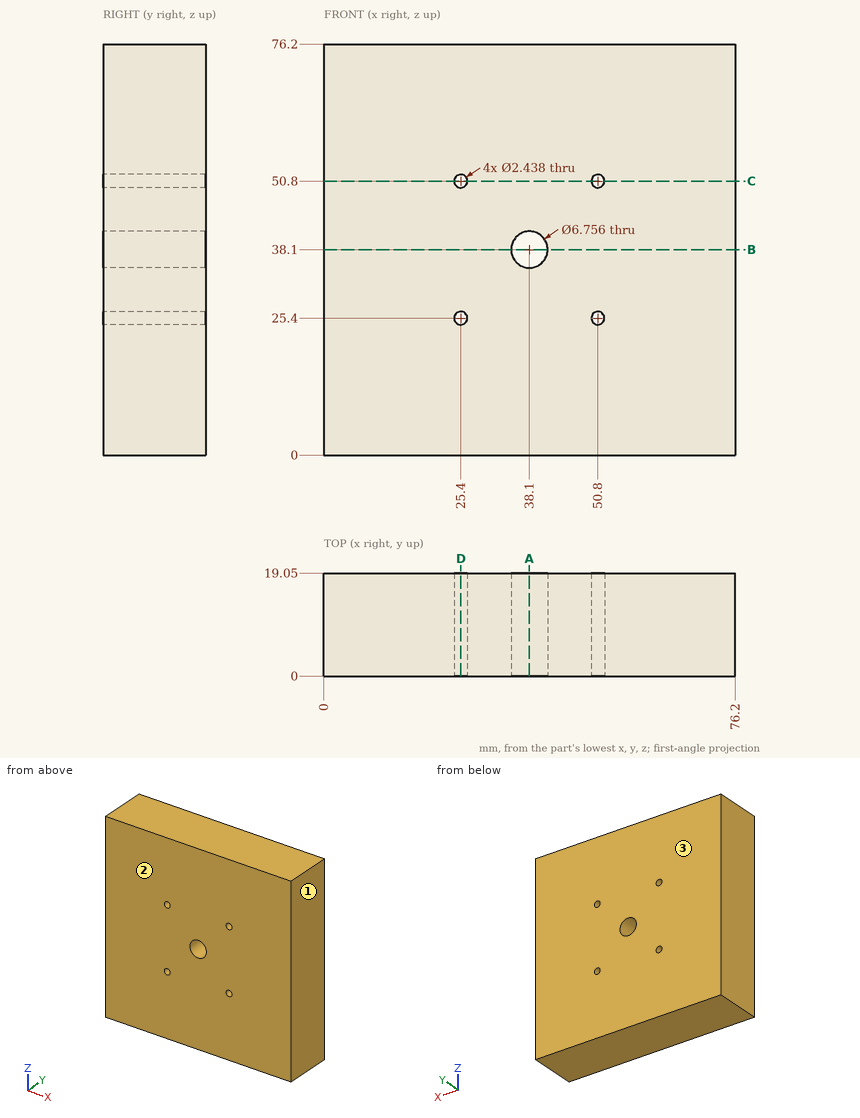
Design review of the part shown in the three views and the two pictorial views. Dimensions are in mm from the part's minimum x, y and z. Coordinates: 2 decimals unless noted, no trailing zeros. Order: outer loops, then holes, each group sorted by start corner. A loop starts at its lowest first (then second) coordinate and runs counter-clockwise, first axis right, second up.
1) Take a section at C-C, the plane z = 50.8. Give the boundary of the cut face in (x, y).
2) Take a section at A-A, the plane x = 38.1. Give the boundary of the cut face in (y, z), and give its area (3 significant figures).
3) Mouldability with a two-part tool opening along Y and no side actions: class the marked faces 1, 2 and 3 as +Y half, -Y half, draft (parallel to the pull), parting line (faces both ways), or undercut.
4) Take a section at D-D, the plane x = 25.4. Give the boundary of the cut face in (y, z).
5) Take a section at B-B, the plane z = 38.1. Give the boundary of the cut face in (x, y), and give its area (3 significant figures).
6) Wall thickness on line 1 along X through (y, z) = (8.75, 50.8); line 2 along X through (y, z) = (3.75, 24.5) (1 decimal): over which ranges is each line inside the solid? List them lowest first.
Returned:
1. outline: (0, 0) - (24.18, 0) - (24.18, 19.05) - (0, 19.05) - close; (26.62, 0) - (49.58, 0) - (49.58, 19.05) - (26.62, 19.05) - close; (52.02, 0) - (76.2, 0) - (76.2, 19.05) - (52.02, 19.05) - close
2. outline: (0, 0) - (19.05, 0) - (19.05, 34.72) - (0, 34.72) - close; (0, 41.48) - (19.05, 41.48) - (19.05, 76.2) - (0, 76.2) - close
2. area: 1,320 mm2
3. face 1: draft
3. face 2: -Y half
3. face 3: +Y half
4. outline: (0, 0) - (19.05, 0) - (19.05, 24.18) - (0, 24.18) - close; (0, 26.62) - (19.05, 26.62) - (19.05, 49.58) - (0, 49.58) - close; (0, 52.02) - (19.05, 52.02) - (19.05, 76.2) - (0, 76.2) - close
5. outline: (0, 0) - (34.72, 0) - (34.72, 19.05) - (0, 19.05) - close; (41.48, 0) - (76.2, 0) - (76.2, 19.05) - (41.48, 19.05) - close
5. area: 1,320 mm2
6. line 1: x = 0 to 24.18, 26.62 to 49.58, 52.02 to 76.2
6. line 2: x = 0 to 24.6, 26.2 to 50, 51.6 to 76.2
